Drawing for the job (mm, zero at the part's lowest x, y, z). A direction names the side the tool comes from. Give positions to 0.01 mm unless a question says otherwise; leave off trailing zeros. Loops run counter-clockwise (first coordinate to the right, second up) from the corner with the lowest first, then second, coordinate; pieces in that order, holes last. Notation, with made-up numbers: (-9.75, -24.5) -> (32.25, -24.5) arc R13 cw to (32.25, -2.5) -> close; hole circle Ø2 at (71.25, 37). An arc over 180 degrees is marked (long way). Use CSV: the item, a comma, the result in double quotes. Start each with the question number.
(1) Cut at C-C on y = 4.5. Write the cut outline in (x, z).
(2) Drill centre lines: probe 1 along X at (y, z) = (10.5, 6.5); probe 2 along Z at (x, y) = (6.35, 8.75); probe 3 along X at (y, z) = (11.85, 6.35). Where is each one in solid material? Low to high.
(3) Cut at D-D on z = 1.5. Write the cut outline in (x, y).
(4) Flat gauge pins, fed straight in: pin 1 (4 mm diameter, centred on x = 6.35, z = 6.35, fed in from -Y); pin 2 (1.5 mm diameter, centred on y = 5.5, z = 1.5, fed in from +X); pin 3 (5 mm diameter, centred on y = 5.5, z = 3.5, fed in from -X); pin 4 (1 mm diameter, centred on x = 7.5, y = 6, fed in from +Z). Where does each tip first touch, or does it go through?
(5) 3-axis set-ups, long thin cutter, end or side, ignore diameter. For the marked faces 1, 2 and 3: which of +Z, -Z, +X, -X, +Y, -Y reach the whole face in a straight line?
(6) Cut at B-B on z = 6. Write the cut outline in (x, y).
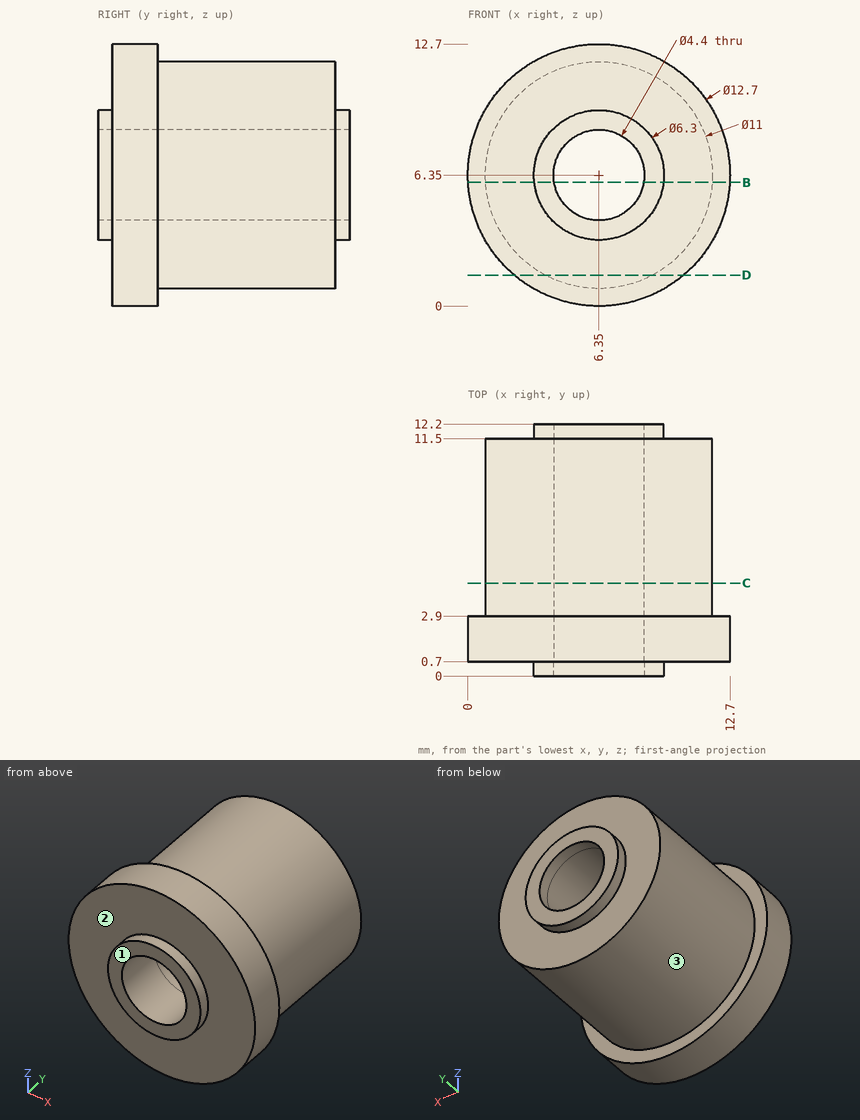
Check result:
1,outline,"circle Ø11 at (6.35, 6.35); hole circle Ø4.4 at (6.35, 6.35)"
2,probe 1,"0.85 to 4.16, 8.54 to 11.85"
2,probe 2,"0.85 to 4.15, 8.55 to 11.85"
2,probe 3,"3.2 to 4.15, 8.55 to 9.5"
3,outline,"(2.25, 0.7) -> (10.45, 0.7) -> (10.45, 2.9) -> (8.94, 2.9) -> (8.94, 11.5) -> (3.76, 11.5) -> (3.76, 2.9) -> (2.25, 2.9) -> close"
4,pin 1,"through"
4,pin 2,"x = 10.02"
4,pin 3,"x = 0.86"
4,pin 4,"z = 11.81"
5,face 1,"+Z, -Z, +X, -X, -Y"
5,face 2,"-Y"
5,face 3,"+Y"
6,outline,"(0.01, 0.7) -> (3.22, 0.7) -> (3.22, 0) -> (4.18, 0) -> (4.18, 12.2) -> (3.22, 12.2) -> (3.22, 11.5) -> (0.86, 11.5) -> (0.86, 2.9) -> (0.01, 2.9) -> close; (8.52, 0) -> (9.48, 0) -> (9.48, 0.7) -> (12.69, 0.7) -> (12.69, 2.9) -> (11.84, 2.9) -> (11.84, 11.5) -> (9.48, 11.5) -> (9.48, 12.2) -> (8.52, 12.2) -> close"
